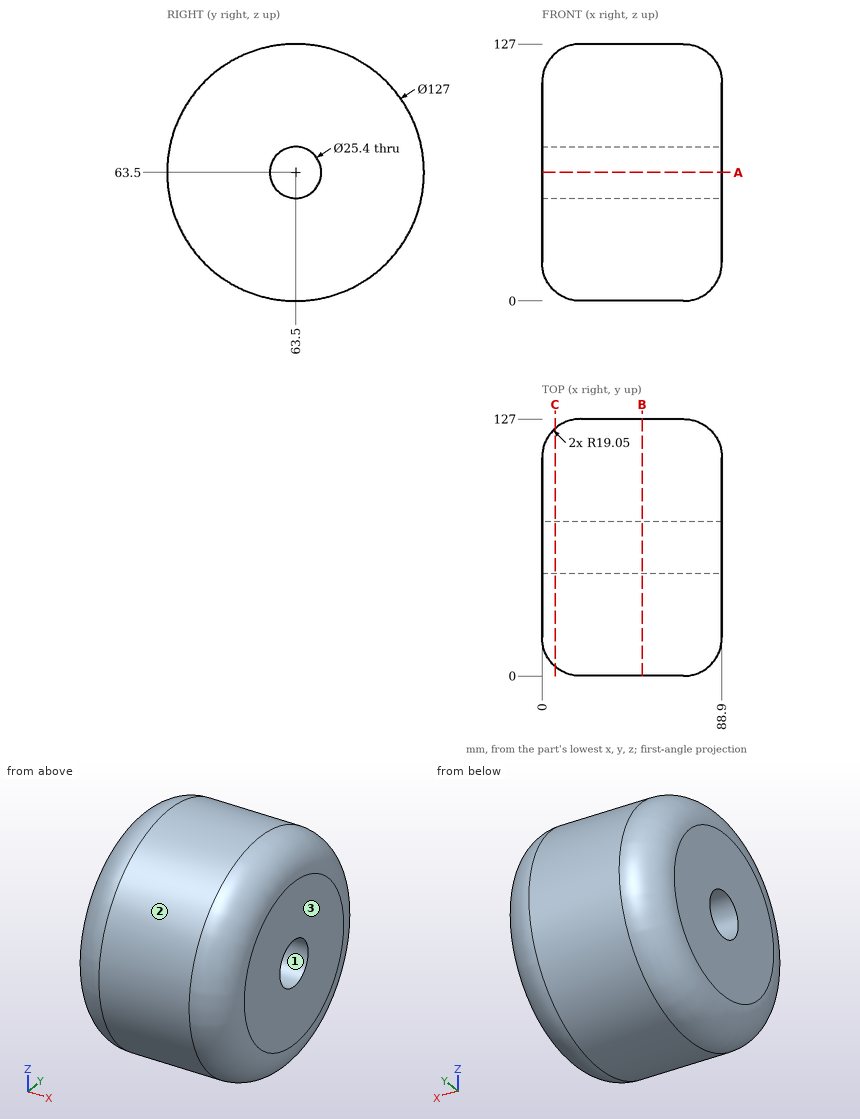
Geometry: see drawing. Coordinates: mm, zero at the bounding-box minimum. Round coordinates to 2 decimals unless told otherwise and drop trailing zeros. Write each loop counter-clockwise with the first axis right and the second up, starting at its lowest first coordinate (ties: lowest second). Pieces come first, ordered by that corner, then holes.
Item 1: Material intervals for L1, parallel to Z at x = 19, y = 63.5; L2, parallel to Y at x = 43, z = 63; L3, parallel to Y at x = 69, z = 59, sorted ascending.
Item 2: Section query C-C (x = 6.5). Return loops of the section in (y, z), plus the area to 3 significant figures.
Item 3: Section query B-B (x = 49.5). Return loops of the section in (y, z), plus the area to 3 significant figures.
Item 4: Section query A-A (z = 63.5). Return loops of the section in (x, y), plus the area to 3 significant figures.
Item 5: Mould query, pull axis Y, two halves, no side actions, for the marked faces 1, 2 and 3. Classes: +Y half, -Y half, draft (parallel to the pull), parting line (faces both ways), or undercut.
Item 6: Pin query (flat end, axial travel): P1, Ø3, axis at x = 53.5, z = 26.5, coming from the -Y side; P2, Ø2, axis at x = 42.5, y = 92.5, coming from the -Z side; P3, Ø1.5, axis at x = 24.5, y = 77, coming from the +Z side. Return the tip coordinate at first contact, or that it passes through.
Completed:
1. L1: z = 0 to 50.8, 76.2 to 127
1. L2: y = 0 to 50.81, 76.19 to 127
1. L3: y = 0.16 to 51.62, 75.38 to 126.84
2. outline: circle Ø117.56 at (63.5, 63.5); hole circle Ø25.4 at (63.5, 63.5)
2. area: 10,300 mm2
3. outline: circle Ø127 at (63.5, 63.5); hole circle Ø25.4 at (63.5, 63.5)
3. area: 12,200 mm2
4. outline: (0, 19.05) arc R19.05 ccw to (19.05, 0) - (69.85, 0) arc R19.05 ccw to (88.9, 19.05) - (88.9, 50.8) - (0, 50.8) - close; (0, 76.2) - (88.9, 76.2) - (88.9, 107.95) arc R19.05 ccw to (69.85, 127) - (19.05, 127) arc R19.05 ccw to (0, 107.95) - close
4. area: 8,720 mm2
5. face 1: undercut
5. face 2: parting line
5. face 3: draft
6. P1: stops at y = 10.85
6. P2: stops at z = 6.51
6. P3: stops at z = 125.71
